```python
from build123d import *

# Parameters (mm, degrees)
SKETCH1_W                       = 44.5
SKETCH1_H                       = 18.7
BOSS_EXTRUDE1_DEPTH             = 139
FILLET1_R                       = 2
SKETCH2_R                       = 1.960015311
SKETCH2_R_2                     = 1.988264752
SKETCH2_R_3                     = 0.918642691
SKETCH2_R_4                     = 0.97117112
SKETCH2_R_5                     = 0.953860003
SKETCH2_R_6                     = 0.951024876
BOSS_EXTRUDE2_DEPTH             = 20
BOSS_EXTRUDE2_DIRECTION_2_REACH = 149.143


with BuildPart() as part:
    # Sketch1 → Boss-Extrude1 (new body)
    with BuildSketch(Plane(origin=(0, 0, 0), x_dir=(1, 0, 0), z_dir=(0, 1, 0))):
        with Locations((22.25, 9.35)):
            Rectangle(SKETCH1_W, SKETCH1_H)
    extrude(amount=BOSS_EXTRUDE1_DEPTH)

    # Fillet1
    fillet1_edges = [part.edges().sort_by_distance(p)[0] for p in [
        (44.5, 139, -9.35),
        (22.25, 139, -18.7),
        (0, 139, -9.35),
        (22.25, 0, -18.7),
        (44.5, 0, -9.35),
        (22.25, 0, 0),
        (0, 0, -9.35),
        (0, 69.5, -18.7),
        (44.5, 69.5, -18.7),
        (44.5, 69.5, 0),
        (0, 69.5, 0),
        (22.25, 139, 0),
    ]]
    fillet(fillet1_edges, radius=FILLET1_R)

    # Sketch2 → Boss-Extrude2 (add)
    with BuildSketch(Plane(origin=(0, 139, 0), x_dir=(1, 0, 0), z_dir=(0, 1, 0))):
        with Locations(Location((42.5, 7.731273805, 0), (0, 0, 270))):
            Circle(SKETCH2_R)
        with Locations(Location((42.5, 12.467660333, 0), (0, 0, 270))):
            Circle(SKETCH2_R_2)
        with Locations(Location((2, 6.327900019, 0), (0, 0, 270))):
            Circle(SKETCH2_R_3)
        with Locations(Location((2, 11.108141978, 0), (0, 0, 270))):
            Circle(SKETCH2_R_4)
        with Locations(Location((2, 13.520190672, 0), (0, 0, 270))):
            Circle(SKETCH2_R_5)
        with Locations(Location((2, 8.827659575, 0), (0, 0, 270))):
            Circle(SKETCH2_R_6)
    extrude(amount=BOSS_EXTRUDE2_DEPTH)

    # Sketch2 → Boss-Extrude2 direction 2 (add, up to next)
    with BuildSketch(Plane(origin=(0, 139, 0), x_dir=(1, 0, 0), z_dir=(0, 1, 0)), mode=Mode.PRIVATE) as boss_extrude2_direction_2_sk1:
        with Locations(Location((42.5, 7.731273805, 0), (0, 0, 270))):
            Circle(SKETCH2_R)
    boss_extrude2_direction_2_tool1 = extrude(boss_extrude2_direction_2_sk1.sketch, amount=-BOSS_EXTRUDE2_DIRECTION_2_REACH, mode=Mode.PRIVATE) - part.part
    # Sketch2 → Boss-Extrude2 direction 2 (add, up to next)
    with BuildSketch(Plane(origin=(0, 139, 0), x_dir=(1, 0, 0), z_dir=(0, 1, 0)), mode=Mode.PRIVATE) as boss_extrude2_direction_2_sk2:
        with Locations(Location((42.5, 12.467660333, 0), (0, 0, 270))):
            Circle(SKETCH2_R_2)
    boss_extrude2_direction_2_tool2 = extrude(boss_extrude2_direction_2_sk2.sketch, amount=-BOSS_EXTRUDE2_DIRECTION_2_REACH, mode=Mode.PRIVATE) - part.part
    # Sketch2 → Boss-Extrude2 direction 2 (add, up to next)
    with BuildSketch(Plane(origin=(0, 139, 0), x_dir=(1, 0, 0), z_dir=(0, 1, 0)), mode=Mode.PRIVATE) as boss_extrude2_direction_2_sk3:
        with Locations(Location((2, 6.327900019, 0), (0, 0, 270))):
            Circle(SKETCH2_R_3)
    boss_extrude2_direction_2_tool3 = extrude(boss_extrude2_direction_2_sk3.sketch, amount=-BOSS_EXTRUDE2_DIRECTION_2_REACH, mode=Mode.PRIVATE) - part.part
    # Sketch2 → Boss-Extrude2 direction 2 (add, up to next)
    with BuildSketch(Plane(origin=(0, 139, 0), x_dir=(1, 0, 0), z_dir=(0, 1, 0)), mode=Mode.PRIVATE) as boss_extrude2_direction_2_sk4:
        with Locations(Location((2, 11.108141978, 0), (0, 0, 270))):
            Circle(SKETCH2_R_4)
    boss_extrude2_direction_2_tool4 = extrude(boss_extrude2_direction_2_sk4.sketch, amount=-BOSS_EXTRUDE2_DIRECTION_2_REACH, mode=Mode.PRIVATE) - part.part
    # Sketch2 → Boss-Extrude2 direction 2 (add, up to next)
    with BuildSketch(Plane(origin=(0, 139, 0), x_dir=(1, 0, 0), z_dir=(0, 1, 0)), mode=Mode.PRIVATE) as boss_extrude2_direction_2_sk5:
        with Locations(Location((2, 13.520190672, 0), (0, 0, 270))):
            Circle(SKETCH2_R_5)
    boss_extrude2_direction_2_tool5 = extrude(boss_extrude2_direction_2_sk5.sketch, amount=-BOSS_EXTRUDE2_DIRECTION_2_REACH, mode=Mode.PRIVATE) - part.part
    # Sketch2 → Boss-Extrude2 direction 2 (add, up to next)
    with BuildSketch(Plane(origin=(0, 139, 0), x_dir=(1, 0, 0), z_dir=(0, 1, 0)), mode=Mode.PRIVATE) as boss_extrude2_direction_2_sk6:
        with Locations(Location((2, 8.827659575, 0), (0, 0, 270))):
            Circle(SKETCH2_R_6)
    boss_extrude2_direction_2_tool6 = extrude(boss_extrude2_direction_2_sk6.sketch, amount=-BOSS_EXTRUDE2_DIRECTION_2_REACH, mode=Mode.PRIVATE) - part.part
    add(boss_extrude2_direction_2_tool1.solids().sort_by_distance((42.5, 139, -7.731274))[0])
    add(boss_extrude2_direction_2_tool2.solids().sort_by_distance((42.5, 139, -12.46766))[0])
    add(boss_extrude2_direction_2_tool3.solids().sort_by_distance((2, 139, -6.3279))[0])
    add(boss_extrude2_direction_2_tool4.solids().sort_by_distance((2, 139, -11.108142))[0])
    add(boss_extrude2_direction_2_tool5.solids().sort_by_distance((2, 139, -13.520191))[0])
    add(boss_extrude2_direction_2_tool6.solids().sort_by_distance((2, 139, -8.82766))[0])


solid = part.part
```
Part model, mm, in its own coordinate system. Round coordinates to 2 decimals unless told otherwise and drop trailing zeros. Write each loop counter-clockwise with the first axis right and the second up, starting at its lowest first coordinate (ties: lowest second). Pieces come first, ordered by that corner, then holes. Notation, with made-up numbers: (19, 63.25) -> (58, 63.25) arc R7 cw to (58, 72.25) -> close; hole circle Ø2 at (82, 43.5). An arc over 180 degrees is marked (long way). Return JSON: item names as keys, results as strings. Group by question number.
Q1. Saw through at B-B on z = -4. Write the cut outline in (x, y).
Q2. Probe L1, parallel to Y at x = 4, z = -6; L2, parallel to Y at x = 28, z = -1.5. List the from-to ranges inside material, lowest first. Write a range as [from, to].
Q3. Saw through at A-A on x = 10. Write the cut outline in (y, z), plus the area to 3 significant figures.
Q4. Mould opens along Z. For faces 1 (the flat face through (43, 159, -8)), 2 (the flat face through (22, 69, -18.7)), 3 (the flat face through (22, 69, 0)) say: pulls with the +Z half, pulls with the -Z half, needs draft (parallel to the pull), parting line crosses it, or undercut.
Answer:
{
 "1": {"outline": "(0, 2) arc R2 ccw to (2, 0) -> (42.5, 0) arc R2 ccw to (44.5, 2) -> (44.5, 137) arc R2 ccw to (42.5, 139) -> (2, 139) arc R2 ccw to (0, 137) -> close"},
 "2": {"L1": "[0, 139]", "L2": "[0.06, 138.94]"},
 "3": {"outline": "(0, -16.7) arc R2 ccw to (2, -18.7) -> (137, -18.7) arc R2 ccw to (139, -16.7) -> (139, -2) arc R2 ccw to (137, 0) -> (2, 0) arc R2 ccw to (0, -2) -> close", "area": "2,600 mm2"},
 "4": {"face 1": "needs draft", "face 2": "pulls with the -Z half", "face 3": "pulls with the +Z half"}
}
